from build123d import *

# Parameters (mm, degrees)
F0_W          = 40
F0_H          = 40
F0_R          = 12.5
F1_DEPTH      = 20
F1_DEPTH_BACK = 20
F2_T1_DEPTH   = 30
F2_T3_DEPTH   = 30
F2_T5_DEPTH   = 30
F2_S9_W       = 5
F2_S9_H       = 5
F2_T10_DEPTH  = 5
F2_S15_W      = 5
F2_S15_H      = 5
F2_T16_DEPTH  = 5
F2_S21_W      = 5
F2_S21_H      = 5
F2_T22_DEPTH  = 5
F2_S27_W      = 5
F2_S27_H      = 5
F2_T28_DEPTH  = 5
F2_S33_W      = 5
F2_S33_H      = 5
F2_T34_DEPTH  = 5
F2_S39_W      = 5
F2_S39_H      = 5
F2_T40_DEPTH  = 5
F2_S45_W      = 5
F2_S45_H      = 5
F2_T46_DEPTH  = 5
F2_S51_W      = 5
F2_S51_H      = 5
F2_T52_DEPTH  = 5


# Not quite as in the source:
# - a fillet or chamfer that OpenCascade refuses, or shapes differently, is made with other operations: its cross-section is extruded or revolved along the edge and cut away or added


with BuildPart() as f1:
    # F0 (on Top) → F1 (new body, two sides)
    with BuildSketch(Plane.XY) as f1_sk:
        Rectangle(F0_W, F0_H)
        Circle(F0_R, mode=Mode.SUBTRACT)
    extrude(amount=F1_DEPTH)
    extrude(f1_sk.sketch, amount=-F1_DEPTH_BACK)

    # F2: fillet of radius 5 on 14 edges, made by hand

    # F2_s2 → F2_t1 (cut)
    with BuildSketch(Plane.XZ.offset(-15)):
        with BuildLine():
            ThreePointArc((20, 15), (18.5355339059, 18.5355339059), (15, 20))
            Line((15, 20), (20, 20))
            Line((20, 20), (20, 15))
        make_face()
        with BuildLine():
            ThreePointArc((-20, 15), (-18.5355339059, 18.5355339059), (-15, 20))
            Line((-15, 20), (-20, 20))
            Line((-20, 20), (-20, 15))
        make_face()
        with BuildLine():
            ThreePointArc((20, -15), (18.5355339059, -18.5355339059), (15, -20))
            Line((15, -20), (20, -20))
            Line((20, -20), (20, -15))
        make_face()
        with BuildLine():
            ThreePointArc((-15, -20), (-18.5355339059, -18.5355339059), (-20, -15))
            Line((-20, -15), (-20, -20))
            Line((-20, -20), (-15, -20))
        make_face()
    extrude(amount=F2_T1_DEPTH, mode=Mode.SUBTRACT)

    # F2_s4 → F2_t3 (cut)
    with BuildSketch(Plane.YZ.offset(-15)):
        with BuildLine():
            ThreePointArc((20, 15), (18.5355339059, 18.5355339059), (15, 20))
            Line((15, 20), (20, 20))
            Line((20, 20), (20, 15))
        make_face()
        with BuildLine():
            ThreePointArc((-15, 20), (-18.5355339059, 18.5355339059), (-20, 15))
            Line((-20, 15), (-20, 20))
            Line((-20, 20), (-15, 20))
        make_face()
        with BuildLine():
            ThreePointArc((15, -20), (18.5355339059, -18.5355339059), (20, -15))
            Line((20, -15), (20, -20))
            Line((20, -20), (15, -20))
        make_face()
        with BuildLine():
            ThreePointArc((-15, -20), (-18.5355339059, -18.5355339059), (-20, -15))
            Line((-20, -15), (-20, -20))
            Line((-20, -20), (-15, -20))
        make_face()
    extrude(amount=F2_T3_DEPTH, mode=Mode.SUBTRACT)

    # F2_s6 → F2_t5 (cut)
    with BuildSketch(Plane.XY.offset(-15)):
        with BuildLine():
            ThreePointArc((-20, 15), (-18.5355339059, 18.5355339059), (-15, 20))
            Line((-15, 20), (-20, 20))
            Line((-20, 20), (-20, 15))
        make_face()
        with BuildLine():
            ThreePointArc((20, 15), (18.5355339059, 18.5355339059), (15, 20))
            Line((15, 20), (20, 20))
            Line((20, 20), (20, 15))
        make_face()
        with BuildLine():
            ThreePointArc((-20, -15), (-18.5355339059, -18.5355339059), (-15, -20))
            Line((-15, -20), (-20, -20))
            Line((-20, -20), (-20, -15))
        make_face()
        with BuildLine():
            ThreePointArc((20, -15), (18.5355339059, -18.5355339059), (15, -20))
            Line((15, -20), (20, -20))
            Line((20, -20), (20, -15))
        make_face()
    extrude(amount=F2_T5_DEPTH, mode=Mode.SUBTRACT)


with BuildPart() as f2_tool8:
    # F2_s9 → F2_t10 (new body)
    with BuildSketch(Plane.YZ.offset(15)):
        with Locations((-17.5, 17.5)):
            Rectangle(F2_S9_W, F2_S9_H)
    extrude(amount=F2_T10_DEPTH)

    # F2_s11 → F2_t12 (revolve, cut)
    with BuildSketch(Plane(origin=(15, -15, 15), x_dir=(0, 0.7071067812, -0.7071067812), z_dir=(0, -0.7071067812, -0.7071067812))):
        with BuildLine():
            ThreePointArc((0, -5), (5, 0), (0, 5))
            Line((0, 5), (0, -5))
        make_face()
    revolve(axis=Axis((15, -15, 15), (1, 0, 0)), mode=Mode.SUBTRACT)


with BuildPart() as f1_1:
    add(f1.part)

    # F2_t7: cut F2_tool8
    add(f2_tool8.part, mode=Mode.SUBTRACT)


with BuildPart() as f2_tool14:
    # F2_s15 → F2_t16 (new body)
    with BuildSketch(Plane.YZ.offset(15)):
        with Locations((17.5, 17.5)):
            Rectangle(F2_S15_W, F2_S15_H)
    extrude(amount=F2_T16_DEPTH)

    # F2_s17 → F2_t18 (revolve, cut)
    with BuildSketch(Plane(origin=(15, 15, 15), x_dir=(0, -0.7071067812, -0.7071067812), z_dir=(0, -0.7071067812, 0.7071067812))):
        with BuildLine():
            ThreePointArc((0, -5), (5, 0), (0, 5))
            Line((0, 5), (0, -5))
        make_face()
    revolve(axis=Axis((15, 15, 15), (1, 0, 0)), mode=Mode.SUBTRACT)


with BuildPart() as f1_2:
    add(f1_1.part)

    # F2_t13: cut F2_tool14
    add(f2_tool14.part, mode=Mode.SUBTRACT)


with BuildPart() as f2_tool20:
    # F2_s21 → F2_t22 (new body)
    with BuildSketch(Plane.YZ.offset(-15)):
        with Locations((17.5, 17.5)):
            Rectangle(F2_S21_W, F2_S21_H)
    extrude(amount=-F2_T22_DEPTH)

    # F2_s23 → F2_t24 (revolve, cut)
    with BuildSketch(Plane(origin=(-15, 15, 15), x_dir=(0, -0.7071067812, -0.7071067812), z_dir=(0, 0.7071067812, -0.7071067812))):
        with BuildLine():
            ThreePointArc((0, -5), (5, 0), (0, 5))
            Line((0, 5), (0, -5))
        make_face()
    revolve(axis=Axis((-15, 15, 15), (-1, 0, 0)), mode=Mode.SUBTRACT)


with BuildPart() as f1_3:
    add(f1_2.part)

    # F2_t19: cut F2_tool20
    add(f2_tool20.part, mode=Mode.SUBTRACT)


with BuildPart() as f2_tool26:
    # F2_s27 → F2_t28 (new body)
    with BuildSketch(Plane.YZ.offset(-15)):
        with Locations((-17.5, 17.5)):
            Rectangle(F2_S27_W, F2_S27_H)
    extrude(amount=-F2_T28_DEPTH)

    # F2_s29 → F2_t30 (revolve, cut)
    with BuildSketch(Plane(origin=(-15, -15, 15), x_dir=(0, 0.7071067812, -0.7071067812), z_dir=(0, 0.7071067812, 0.7071067812))):
        with BuildLine():
            ThreePointArc((0, -5), (5, 0), (0, 5))
            Line((0, 5), (0, -5))
        make_face()
    revolve(axis=Axis((-15, -15, 15), (-1, 0, 0)), mode=Mode.SUBTRACT)


with BuildPart() as f1_4:
    add(f1_3.part)

    # F2_t25: cut F2_tool26
    add(f2_tool26.part, mode=Mode.SUBTRACT)


with BuildPart() as f2_tool32:
    # F2_s33 → F2_t34 (new body)
    with BuildSketch(Plane.XY.offset(-15)):
        with Locations((-17.5, 17.5)):
            Rectangle(F2_S33_W, F2_S33_H)
    extrude(amount=-F2_T34_DEPTH)

    # F2_s35 → F2_t36 (revolve, cut)
    with BuildSketch(Plane(origin=(-15, 15, -15), x_dir=(0.7071067812, -0.7071067812, 0), z_dir=(0.7071067812, 0.7071067812, 0))):
        with BuildLine():
            ThreePointArc((0, -5), (5, 0), (0, 5))
            Line((0, 5), (0, -5))
        make_face()
    revolve(axis=Axis((-15, 15, -15), (0, 0, -1)), mode=Mode.SUBTRACT)


with BuildPart() as f1_5:
    add(f1_4.part)

    # F2_t31: cut F2_tool32
    add(f2_tool32.part, mode=Mode.SUBTRACT)


with BuildPart() as f2_tool38:
    # F2_s39 → F2_t40 (new body)
    with BuildSketch(Plane.YZ.offset(15)):
        with Locations((17.5, -17.5)):
            Rectangle(F2_S39_W, F2_S39_H)
    extrude(amount=F2_T40_DEPTH)

    # F2_s41 → F2_t42 (revolve, cut)
    with BuildSketch(Plane(origin=(15, 15, -15), x_dir=(0, -0.7071067812, 0.7071067812), z_dir=(0, 0.7071067812, 0.7071067812))):
        with BuildLine():
            ThreePointArc((0, -5), (5, 0), (0, 5))
            Line((0, 5), (0, -5))
        make_face()
    revolve(axis=Axis((15, 15, -15), (1, 0, 0)), mode=Mode.SUBTRACT)


with BuildPart() as f1_6:
    add(f1_5.part)

    # F2_t37: cut F2_tool38
    add(f2_tool38.part, mode=Mode.SUBTRACT)


with BuildPart() as f2_tool44:
    # F2_s45 → F2_t46 (new body)
    with BuildSketch(Plane.YZ.offset(15)):
        with Locations((-17.5, -17.5)):
            Rectangle(F2_S45_W, F2_S45_H)
    extrude(amount=F2_T46_DEPTH)

    # F2_s47 → F2_t48 (revolve, cut)
    with BuildSketch(Plane(origin=(15, -15, -15), x_dir=(0, 0.7071067812, 0.7071067812), z_dir=(0, 0.7071067812, -0.7071067812))):
        with BuildLine():
            ThreePointArc((0, -5), (5, 0), (0, 5))
            Line((0, 5), (0, -5))
        make_face()
    revolve(axis=Axis((15, -15, -15), (1, 0, 0)), mode=Mode.SUBTRACT)


with BuildPart() as f1_7:
    add(f1_6.part)

    # F2_t43: cut F2_tool44
    add(f2_tool44.part, mode=Mode.SUBTRACT)


with BuildPart() as f2_tool50:
    # F2_s51 → F2_t52 (new body)
    with BuildSketch(Plane.XY.offset(-15)):
        with Locations((-17.5, -17.5)):
            Rectangle(F2_S51_W, F2_S51_H)
    extrude(amount=-F2_T52_DEPTH)

    # F2_s53 → F2_t54 (revolve, cut)
    with BuildSketch(Plane(origin=(-15, -15, -15), x_dir=(0.7071067812, 0.7071067812, 0), z_dir=(-0.7071067812, 0.7071067812, 0))):
        with BuildLine():
            ThreePointArc((0, -5), (5, 0), (0, 5))
            Line((0, 5), (0, -5))
        make_face()
    revolve(axis=Axis((-15, -15, -15), (0, 0, -1)), mode=Mode.SUBTRACT)


with BuildPart() as f1_8:
    add(f1_7.part)

    # F2_t49: cut F2_tool50
    add(f2_tool50.part, mode=Mode.SUBTRACT)

    # F2_s55 → F2_t56 (revolve, cut)
    with BuildSketch(Plane.XZ):
        with BuildLine():
            ThreePointArc((12.5, 15), (13.9644660941, 18.5355339059), (17.5, 20))
            Line((17.5, 20), (12.5, 20))
            Line((12.5, 20), (12.5, 15))
        make_face()
    revolve(axis=Axis((0, 0, 20), (0, 0, 1)), mode=Mode.SUBTRACT)

    # F2_s57 → F2_t58 (revolve, cut)
    with BuildSketch(Plane.XZ):
        with BuildLine():
            ThreePointArc((17.5, -20), (13.9644660941, -18.5355339059), (12.5, -15))
            Line((12.5, -15), (12.5, -20))
            Line((12.5, -20), (17.5, -20))
        make_face()
    revolve(axis=Axis((0, 0, -20), (0, 0, 1)), mode=Mode.SUBTRACT)


solid = f1_8.part
The model under review builds one solid part; all positions refer to its coordinate system, in mm. Coordinates: 2 decimals unless noted, no trailing zeros. Loops run counter-clockwise (first coordinate to the right, second up) from the corner with the lowest first, then second, coordinate; pieces in that order, holes last. Notation, with made-up numbers: M -26,13 L 20,13 A14 cw 20,20 Z; hole C -22.5,-8 d6. An arc over 180 degrees is marked long. Put each result on its own line as item: value. Start each with the question number.
Q1. The part is to be moulded in two halves that separate along Y. For faces 1 (the cylindrical face through (0, -18, 19)), 2 (the flat face through (13, -13, -20)), 3 (the cylindrical face through (11.923, 3.755, -0.21)), say which applies: +Y half, -Y half, draft (parallel to the pull), parting line (faces both ways), or undercut.
Q2. Add section A-A (z = 3.5). Write out the cut boundary in (x, y), and give its area (3 significant figures).
Q3. Wall thickness on line 1 (Y direction, x = 0, z = 9); line 2 (X direction, y = -8, z = -14.5); line 3 (X direction, y = 4, z = -11): over which ranges is each line inside the solid? List them lowest first.
Q4. Add section D-D (y = 17). Write out the cut boundary in (x, z).
Q5. Clearance check with a flat-ended pin moving along its axis: pin 1 (8 mm diameter, centred on x = -8, y = 4.5, fed in from +Z). State where the tip first meets the part, or that it passes through.
Q6. Add section B-B (y = 0). Write out the cut boundary in (x, z), and give its area (3 significant figures).
Answers:
1. face 1: -Y half
1. face 2: draft
1. face 3: undercut
2. outline: M -20,-15 A5 ccw -15,-20 L 15,-20 A5 ccw 20,-15 L 20,15 A5 ccw 15,20 L -15,20 A5 ccw -20,15 Z; hole C 0,0 d25
2. area: 1,090 mm^2
3. line 1: y = -20 to -12.5, 12.5 to 20
3. line 2: x = -20 to -9.6, 9.6 to 20
3. line 3: x = -20 to -11.84, 11.84 to 20
4. outline: M -19.58,-15 A4.58 ccw -15,-19.58 L 15,-19.58 A4.58 ccw 19.58,-15 L 19.58,15 A4.58 ccw 15,19.58 L -15,19.58 A4.58 ccw -19.58,15 Z
5. pin 1: stops at z = 17.52
6. outline: M -20,-15 A5 ccw -16.25,-19.84 A5 ccw -12.5,-15 L -12.5,15 A5 ccw -16.25,19.84 A5 ccw -20,15 Z; M 12.5,-15 A5 ccw 16.25,-19.84 A5 ccw 20,-15 L 20,15 A5 ccw 16.25,19.84 A5 ccw 12.5,15 Z
6. area: 558 mm^2
